```python
from build123d import *

# Parameters (mm, degrees)
BOSS_EXTRUDE1_DEPTH = 9
SKETCH2_R           = 2.75
CUT_EXTRUDE1_DEPTH  = 10


with BuildPart() as part:
    # Sketch1 → Boss-Extrude1 (new body)
    with BuildSketch(Plane(origin=(0, 0, 0), x_dir=(1, 0, 0), z_dir=(0, 1, 0))):
        Polygon((-35, 118.5), (-50, 118.5), (-50, -118.5), (-35, -118.5), (-35, -127.5), (-15, -127.5), (-15, -118.5), (15, -118.5), (15, -127.5), (35, -127.5), (35, -118.5), (50, -118.5), (50, 118.5), (35, 118.5), (35, 109.5), (15, 109.5), (15, 118.5), (-15, 118.5), (-15, 109.5), (-35, 109.5), align=None)
    extrude(amount=BOSS_EXTRUDE1_DEPTH)

    # Sketch2 → Cut-Extrude1 (cut)
    with BuildSketch(Plane(origin=(0, 9, 0), x_dir=(1, 0, 0), z_dir=(0, 1, 0))):
        with Locations(Location((-45, -111.5, 0), (0, 0, 270))):
            Circle(SKETCH2_R)
        with Locations(Location((-13, -111.5, 0), (0, 0, 270))):
            Circle(SKETCH2_R)
        with Locations(Location((13, -111.5, 0), (0, 0, 270))):
            Circle(SKETCH2_R)
        with Locations(Location((45, -111.5, 0), (0, 0, 270))):
            Circle(SKETCH2_R)
        with Locations(Location((-45, 102.5, 0), (0, 0, 270))):
            Circle(SKETCH2_R)
        with Locations(Location((-13, 102.5, 0), (0, 0, 270))):
            Circle(SKETCH2_R)
        with Locations(Location((13, 102.5, 0), (0, 0, 270))):
            Circle(SKETCH2_R)
        with Locations(Location((45, 102.5, 0), (0, 0, 270))):
            Circle(SKETCH2_R)
    extrude(amount=-CUT_EXTRUDE1_DEPTH, mode=Mode.SUBTRACT)


solid = part.part
```
Part model, mm, in its own coordinate system. A direction names the side the tool comes from. Round coordinates to 2 decimals unless told otherwise and drop trailing zeros. Write each loop counter-clockwise with the first axis right and the second up, starting at its lowest first coordinate (ties: lowest second). Pieces come first, ordered by that corner, then holes.
Item 1: Cut at B-B, the plane z = -102.5. Give the cut face in (x, y), plus the area to 3 significant figures.
Results:
outline: (-50, 0) - (-47.75, 0) - (-47.75, 9) - (-50, 9) - close; (-42.25, 0) - (-15.75, 0) - (-15.75, 9) - (-42.25, 9) - close; (-10.25, 0) - (10.25, 0) - (10.25, 9) - (-10.25, 9) - close; (15.75, 0) - (42.25, 0) - (42.25, 9) - (15.75, 9) - close; (47.75, 0) - (50, 0) - (50, 9) - (47.75, 9) - close
area: 702 mm2
Item 2: Cut at D-D, the plane x = -4.5. Give the cut face in (y, z), plus the area to 3 significant figures.
Results:
outline: (0, -118.5) - (9, -118.5) - (9, 118.5) - (0, 118.5) - close
area: 2,130 mm2
Item 3: Cut at C-C, the plane y = 1.75. Count the separate pieces of the cut face and the enclosed holes in it, plus the area to 3 significant figures.
Results:
separate pieces: 1
enclosed holes: 8
area: 23,500 mm2
Item 4: Which spindle directions (+Z, -Z, +X, -X, +Y, -Y) get a long thin tool onto all of the face, cutting with end or side? Do faces 1 (the flat face through (35, 4, -114)), 2 (the flat face through (-35, 4, 123)), 3 (the flat face through (15, 4, 123)). Say none if no direction does.
Results:
face 1: -Z, +Y, -Y
face 2: +Z, -X, +Y, -Y
face 3: +Z, +Y, -Y
Item 5: Cut at A-A, the plane x = -45. Give the cut face in (y, z), plus the area to 3 significant figures.
Results:
outline: (0, -118.5) - (9, -118.5) - (9, -105.25) - (0, -105.25) - close; (0, -99.75) - (9, -99.75) - (9, 108.75) - (0, 108.75) - close; (0, 114.25) - (9, 114.25) - (9, 118.5) - (0, 118.5) - close
area: 2,030 mm2
Item 6: Probe L1, parallel to X at y = 5, z = 111.5; L2, parallel to Z at x = 17, y = 1.25; L3, parallel to Z at x = 11, y = 5. List the from-to ranges inside material, lowest first.
Results:
L1: x = -50 to -47.75, -42.25 to -15.75, -10.25 to 10.25, 15.75 to 42.25, 47.75 to 50
L2: z = -109.5 to 127.5
L3: z = -118.5 to -104.39, -100.61 to 109.61, 113.39 to 118.5
Item 7: Drop flat-ended pins along their axis: pin 1 Ø4.5 at (x, y) = (46, 6.5) entering from +Z; pin 2 Ø4.5 at (x, y) = (-24.5, 3) entering from -Z. Give the stop position or say it passes through.
Results:
pin 1: stops at z = 118.5
pin 2: stops at z = -109.5
Item 8: Two-plate mould, pull along Z, no slides. Class faces 4 (the flat face through (-25, 4, 127.5)), 5 (the flat face through (25, 4, -109.5)), 6 (the cylindrical face through (46.859, 4.563, 109.473)), 7 (the cylindrical face through (13.121, 4.563, -105.247)): +Z half, -Z half, draft (parallel to the pull), parting line (faces both ways), or undercut.
Results:
face 4: +Z half
face 5: -Z half
face 6: undercut
face 7: undercut
